```python
from build123d import *

# Parameters (mm, degrees)
SKETCH1_W                                            = 18.8
SKETCH1_H                                            = 11.6
BOSS_EXTRUDE1_DEPTH                                  = 11.5
SKETCH2_W                                            = 34.15
SKETCH2_H                                            = 11.8
BOSS_EXTRUDE2_DEPTH                                  = 2.5
BOSS_EXTRUDE3_DEPTH                                  = 2.5
FILLET1_R                                            = 1.5
FILLET2_R                                            = 1
CSK_FOR_M3_HEX_SOCKET_COUNTERSUNK_HEAD_S_D           = 3.1
CSK_FOR_M3_HEX_SOCKET_COUNTERSUNK_HEAD_S_CSINK_D     = 6.7
CSK_FOR_M3_HEX_SOCKET_COUNTERSUNK_HEAD_S_CSINK_ANGLE = 90
FILLET3_R                                            = 3
FILLET4_R                                            = 1
CUT_EXTRUDE1_DEPTH                                   = 2
SKETCH7_W                                            = 6.4
SKETCH7_H                                            = 6.2
CUT_EXTRUDE2_DEPTH                                   = 2
FILLET5_R                                            = 1.5
SKETCH8_R                                            = 2.1
BOSS_EXTRUDE4_DEPTH                                  = 6.5
F_3_0MM_DOWEL_HOLE1_D                                = 3
F_3_0MM_DOWEL_HOLE1_DEPTH                            = 3.3
F_3_0MM_DOWEL_HOLE1_TIP                              = 0.901290929
SKETCH11_W                                           = 3.39233295
SKETCH11_H                                           = 4.331282249
SKETCH11_W_2                                         = 2.756270522
SKETCH11_H_2                                         = 5.335422798
CUT_EXTRUDE3_DEPTH                                   = 3.25
FILLET6_R                                            = 0.2
CUT_EXTRUDE6_DEPTH                                   = 8.8
SKETCH13_R                                           = 2
CUT_EXTRUDE7_DEPTH                                   = 0.1
SKETCH14_R                                           = 1.75
CUT_EXTRUDE8_DEPTH                                   = 12
SKETCH15_W                                           = 0.583333334
SKETCH15_H                                           = 1.211538462
BOSS_EXTRUDE5_DEPTH                                  = 0.1
BOSS_EXTRUDE6_DEPTH                                  = 0.1


with BuildPart() as part:
    # Sketch1 → Boss-Extrude1 (new body)
    with BuildSketch(Plane.XY):
        Rectangle(SKETCH1_W, SKETCH1_H)
    extrude(amount=-BOSS_EXTRUDE1_DEPTH)

    # Sketch2 → Boss-Extrude2 (add)
    with BuildSketch(Plane.XY):
        Rectangle(SKETCH2_W, SKETCH2_H)
    extrude(amount=BOSS_EXTRUDE2_DEPTH)

    # Sketch3 → Boss-Extrude3 (add)
    with BuildSketch(Plane.XY):
        Polygon((-10, 8.3), (-13.075, 5.9), (-13.075, -5.9), (-9.036144578, -7.5), (9.036144578, -7.5), (13.075, -5.9), (13.075, 5.9), (10, 8.3), align=None)
    extrude(amount=BOSS_EXTRUDE3_DEPTH)

    # Fillet1
    fillet1_edges = [part.edges().sort_by_distance(p)[0] for p in [
        (-17.075, 5.9, 1.25),
        (-17.075, -5.9, 1.25),
        (17.075, -5.9, 1.25),
        (17.075, 5.9, 1.25),
    ]]
    fillet(fillet1_edges, radius=FILLET1_R)

    # Fillet2
    fillet2_edges = [part.edges().sort_by_distance(p)[0] for p in [
        (10, 8.3, 1.25),
        (-10, 8.3, 1.25),
        (-13.075, 5.9, 1.25),
        (-13.075, -5.9, 1.25),
        (-9.036144578, -7.5, 1.25),
        (9.036144578, -7.5, 1.25),
        (13.075, -5.9, 1.25),
        (13.075, 5.9, 1.25),
    ]]
    fillet(fillet2_edges, radius=FILLET2_R)

    # CSK for M3 Hex Socket Countersunk Head Screw1 (through all)
    with Locations(Plane.XY.offset(2.5)):
        with Locations((-12.5, 0), (12.5, 0)):
            CounterSinkHole(CSK_FOR_M3_HEX_SOCKET_COUNTERSUNK_HEAD_S_D / 2, CSK_FOR_M3_HEX_SOCKET_COUNTERSUNK_HEAD_S_CSINK_D / 2, counter_sink_angle=CSK_FOR_M3_HEX_SOCKET_COUNTERSUNK_HEAD_S_CSINK_ANGLE)

    # Fillet3
    fillet3_edges = [part.edges().sort_by_distance(p)[0] for p in [
        (9.4, 5.8, -5.75),
        (9.4, -5.8, -5.75),
    ]]
    fillet(fillet3_edges, radius=FILLET3_R)

    # Fillet4
    fillet4_edges = [part.edges().sort_by_distance(p)[0] for p in [
        (-9.4, 5.8, -5.75),
        (-9.4, -5.8, -5.75),
    ]]
    fillet(fillet4_edges, radius=FILLET4_R)

    # Sketch6 → Cut-Extrude1 (cut)
    with BuildSketch(Plane(origin=(0, 0, -7), x_dir=(-1, 0, 0), z_dir=(0, 0, -1))):
        with BuildLine():
            Line((-6.4, -6.7), (8.4, -6.7))
            ThreePointArc((8.4, -6.7), (9.743502884, -6.143502884), (10.3, -4.8))
            Line((10.3, -4.8), (10.3, 4.8))
            ThreePointArc((10.3, 4.8), (9.743502884, 6.143502884), (8.4, 6.7))
            Line((8.4, 6.7), (-6.4, 6.7))
            ThreePointArc((-6.4, 6.7), (-9.157716447, 5.557716447), (-10.3, 2.8))
            Line((-10.3, 2.8), (-10.3, -2.8))
            ThreePointArc((-10.3, -2.8), (-9.157716447, -5.557716447), (-6.4, -6.7))
        make_face()
        with BuildLine():
            Line((-6.4, -4.55), (8.15, -4.55))
            Line((8.15, -4.55), (8.15, 4.55))
            Line((8.15, 4.55), (-6.4, 4.55))
            ThreePointArc((-6.4, 4.55), (-7.637436867, 4.037436867), (-8.15, 2.8))
            Line((-8.15, 2.8), (-8.15, -2.8))
            ThreePointArc((-8.15, -2.8), (-7.637436867, -4.037436867), (-6.4, -4.55))
        make_face(mode=Mode.SUBTRACT)
    extrude(amount=CUT_EXTRUDE1_DEPTH, mode=Mode.SUBTRACT)

    # Sketch7 → Cut-Extrude2 (cut)
    with BuildSketch(Plane(origin=(0, 0, -11.5), x_dir=(-1, 0, 0), z_dir=(0, 0, -1))):
        with Locations((-3.5, 0)):
            Rectangle(SKETCH7_W, SKETCH7_H)
        with Locations((3.5, 0)):
            Rectangle(SKETCH7_W, SKETCH7_H)
    extrude(amount=-CUT_EXTRUDE2_DEPTH, mode=Mode.SUBTRACT)

    # Fillet5
    fillet5_edges = [part.edges().sort_by_distance(p)[0] for p in [
        (6.7, -3.1, -10.5),
        (6.7, 3.1, -10.5),
    ]]
    fillet(fillet5_edges, radius=FILLET5_R)

    # Sketch8 → Boss-Extrude4 (add)
    with BuildSketch(Plane(origin=(0, 0, -9.5), x_dir=(-1, 0, 0), z_dir=(0, 0, -1))):
        with Locations((-3.6, 0)):
            Circle(SKETCH8_R)
        with Locations((3.6, 0)):
            Circle(SKETCH8_R)
    extrude(amount=BOSS_EXTRUDE4_DEPTH)

    # Ø3.0mm Dowel Hole1
    with Locations(Plane(origin=(0, 0, -16), x_dir=(-1, 0, 0), z_dir=(0, 0, -1))):
        with Locations((-3.6, 0), (3.6, 0)):
            Hole(F_3_0MM_DOWEL_HOLE1_D / 2, depth=F_3_0MM_DOWEL_HOLE1_DEPTH)
            with Locations((0, 0, -(F_3_0MM_DOWEL_HOLE1_DEPTH + F_3_0MM_DOWEL_HOLE1_TIP / 2))):  # 118° drill point
                Cone(0, F_3_0MM_DOWEL_HOLE1_D / 2, F_3_0MM_DOWEL_HOLE1_TIP, mode=Mode.SUBTRACT)

    # Sketch11 → Cut-Extrude3 (cut, symmetric)
    with BuildSketch(Plane(origin=(0, 0, 0), x_dir=(1, 0, 0), z_dir=(0, 1, 0))):
        with Locations((-5.296166475, 15.165641125)):
            Rectangle(SKETCH11_W, SKETCH11_H)
        with Locations((4.978135261, 15.667711399)):
            Rectangle(SKETCH11_W_2, SKETCH11_H_2)
    extrude(amount=CUT_EXTRUDE3_DEPTH, both=True, mode=Mode.SUBTRACT)

    # Fillet6
    fillet6_edges = [part.edges().sort_by_distance(p)[0] for p in [
        (-3.6, 1.8, -13),
        (-3.6, -1.8, -13),
        (-3.6, 1.8, -16),
        (-3.6, -1.8, -16),
        (3.6, 1.8, -13),
        (3.6, -1.8, -13),
        (3.6, -1.8, -16),
        (3.6, 1.8, -16),
    ]]
    fillet(fillet6_edges, radius=FILLET6_R)

    # Sketch12 → Cut-Extrude6 (cut)
    with BuildSketch(Plane.XY.offset(2.5)):
        with BuildLine():
            Line((5.9, -4.5), (-8.4, -4.5))
            Line((-8.4, -4.5), (-8.4, 4.5))
            Line((-8.4, 4.5), (5.9, 4.5))
            ThreePointArc((5.9, 4.5), (7.667766953, 3.767766953), (8.4, 2))
            Line((8.4, 2), (8.4, -2))
            ThreePointArc((8.4, -2), (7.667766953, -3.767766953), (5.9, -4.5))
        make_face()
        with BuildLine():
            Line((3.65, -3.15), (-6.8, -3.15))
            Line((-6.8, -3.15), (-6.8, 3.15))
            Line((-6.8, 3.15), (-1, 3.15))
            Line((-1, 3.15), (-1, 1.95))
            Line((-1, 1.95), (1, 1.95))
            Line((1, 1.95), (1, 3.15))
            Line((1, 3.15), (3.65, 3.15))
            ThreePointArc((3.65, 3.15), (6.8, 0), (3.65, -3.15))
        make_face(mode=Mode.SUBTRACT)
    extrude(amount=-CUT_EXTRUDE6_DEPTH, mode=Mode.SUBTRACT)

    # Sketch13 → Cut-Extrude7 (cut)
    with BuildSketch(Plane.XY.offset(2.5)):
        with Locations((-3.6, 0)):
            Circle(SKETCH13_R)
        with Locations((3.6, 0)):
            Circle(SKETCH13_R)
    extrude(amount=-CUT_EXTRUDE7_DEPTH, mode=Mode.SUBTRACT)

    # Sketch14 → Cut-Extrude8 (cut)
    with BuildSketch(Plane.XY.offset(2.5)):
        with Locations((-3.6, 0)):
            Circle(SKETCH14_R)
        with Locations((3.6, 0)):
            Circle(SKETCH14_R)
    extrude(amount=-CUT_EXTRUDE8_DEPTH, mode=Mode.SUBTRACT)

    # Sketch15 → Boss-Extrude5 (add)
    with BuildSketch(Plane(origin=(9.4, 0, 0), x_dir=(0, 0, -1), z_dir=(1, 0, 0))):
        with Locations((10.278846154, -0.201923077)):
            Rectangle(SKETCH15_W, SKETCH15_H)
    extrude(amount=BOSS_EXTRUDE5_DEPTH)

    # Sketch16 → Boss-Extrude6 (add)
    with BuildSketch(Plane.ZY.offset(9.4)):
        Polygon((-10.560064901, -0.314102564), (-11.412629003, -0.314102564), (-11.412629003, 0.269230769), (-10.560064901, 0.269230769), (-10.560064901, 1.166666667), (-9.976731567, 1.166666667), (-9.976731567, 0.269230769), (-9.124167465, 0.269230769), (-9.124167465, -0.314102564), (-9.976731567, -0.314102564), (-9.976731567, -1.211538462), (-10.560064901, -1.211538462), align=None)
    extrude(amount=BOSS_EXTRUDE6_DEPTH)


solid = part.part
```
The model under review builds one solid part; all positions refer to its coordinate system, in mm. A direction names the side the tool comes from. Coordinates: 2 decimals unless noted, no trailing zeros. Write each loop counter-clockwise with the first axis right and the second up, starting at its lowest first coordinate (ties: lowest second). Pieces come first, ordered by that corner, then holes.
1) We need section B-B on z = -7.5. State the section outline as (x, y) points, then the cut area to 3 significant figures.
2) The part is to be moulded in two halves that separate along Z. For faces 4 (the face through (-3.34, 0.011, -11.955)), 5 (the face through (7.651, -4.024, -7.986)), 6 (the face through (7.687, -3.748, -1.838)), say which applies: pulls with the +Z half, pulls with the -Z half, needs draft (parallel to the pull), parting line crosses it, or undercut.
3) We need section A-A on z = -1.5. State the section outline as (x, y) points, then the cut area to 3 significant figures.
4) We need section C-C on y = -3.75. State the section outline as (x, z) points (3 decimals).
5) To check wall thickness, follow probe 1 along Y at (x, z) = (3.6, -4); probe 2 along Y at (x, z) = (-1.5, -1). State the ranges of each line that lie inside material, in increasing order.
6) Clearance check with flat-ended pins moving along their axes: pin 1 Ø1.6 at (x, z) = (3, -10) entering from +Y; pin 2 Ø10 at (x, z) = (8, -13.5) entering from -Y; pin 3 Ø0.6 at (y, z) = (3, -1) entering from -X. State where each tip first meets the part, or that it passes through.
7) Machinability: for faces 1 (the face through (-1, 5.8, -10)), 2 (the face through (0, -5, -7)), 3 (the face through (-1, 4.5, -2)), which of the approach directions +Z, -Z, +X, -X, +Y, -Y give a long, thin tool a straight path to every point of the face, cutting with its end or side? Answer none if there is none.
Answer list:
1. outline: (-8.15, -4.55) - (6.4, -4.55) arc R1.75 ccw to (8.15, -2.8) - (8.15, 2.8) arc R1.75 ccw to (6.4, 4.55) - (-8.15, 4.55) - close; hole circle Ø3.5 at (-3.6, 0); hole circle Ø3.5 at (3.6, 0)
1. area: 128 mm2
2. face 4: pulls with the -Z half
2. face 5: undercut
2. face 6: needs draft
3. outline: (-9.4, -4.8) arc R1 ccw to (-8.4, -5.8) - (6.4, -5.8) arc R3 ccw to (9.4, -2.8) - (9.4, 2.8) arc R3 ccw to (6.4, 5.8) - (-8.4, 5.8) arc R1 ccw to (-9.4, 4.8) - close; (-6.8, -3.15) - (3.65, -3.15) arc R3.15 ccw to (3.65, 3.15) - (1, 3.15) - (1, 1.95) - (-1, 1.95) - (-1, 3.15) - (-6.8, 3.15) - close; hole (-8.4, -4.5) - (5.9, -4.5) arc R2.5 ccw to (8.4, -2) - (8.4, 2) arc R2.5 ccw to (5.9, 4.5) - (-8.4, 4.5) - close; hole circle Ø3.5 at (-3.6, 0); hole circle Ø3.5 at (3.6, 0)
3. area: 125 mm2
4. outline: (-17.075, 0) - (-9.4, 0) - (-9.4, -7) - (-8.15, -7) - (-8.15, -9) - (-9.4, -9) - (-9.4, -11.5) - (9.246, -11.5) - (9.246, -9) - (7.87, -9) - (7.87, -7) - (9.246, -7) - (9.246, 0) - (17.075, 0) - (17.075, 2.5) - (7.685, 2.5) - (7.685, -6.3) - (-8.4, -6.3) - (-8.4, 2.5) - (-17.075, 2.5) - close
5. probe 1: y = -5.8 to -4.5, -3.15 to -1.75, 1.75 to 3.15, 4.5 to 5.8
5. probe 2: y = -5.8 to -4.5, -3.15 to 3.15, 4.5 to 5.8
6. pin 1: stops at y = 5.8
6. pin 2: stops at y = -5.8
6. pin 3: stops at x = -9.4
7. face 1: -Z, +X, -X, +Y
7. face 2: none
7. face 3: +Z
